The drawing under review shows one solid part. Ordinate dimensions are in mm from its lowest x, y, z. Coordinates: 2 decimals unless noted, no trailing zeros. Loops run counter-clockwise (first coordinate to the right, second up) from the corner with the lowest first, then second, coordinate; pieces in that order, holes last. Notation, with made-up numbers: (-39.75, 74.5) -> (4.25, 74.5) arc R10 ccw to (4.25, 81.5) -> close; hole circle Ø9 at (4, 45). An arc over 180 degrees is marked (long way). Use a Markdown table: item, result.
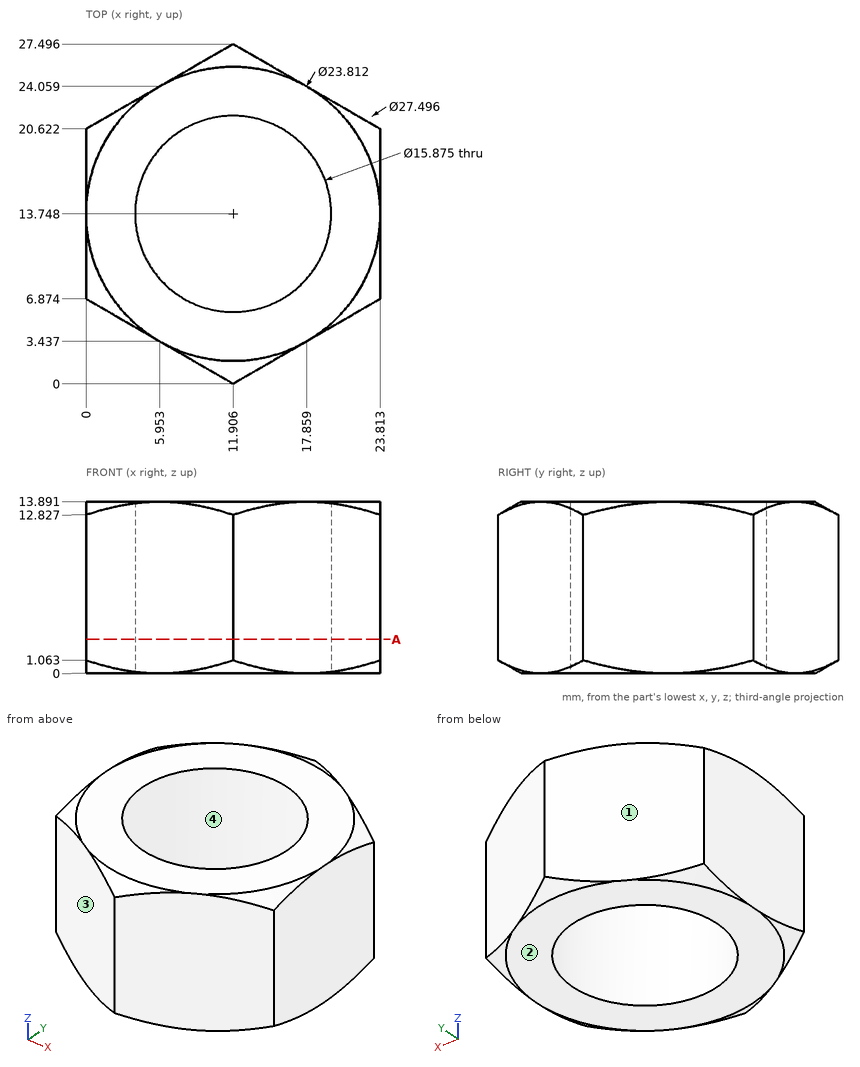
(1) For pin 1 Ø8 at (x, z) = (4, 6.5) entering from -Y (1 decimal); pin 2 Ø4 at (x, y) = (21, 16.5) entering from -Z; pin 3 Ø5 at (x, z) = (20, 12.5) entering from -Y; pin 4 Ø3 at (x, z) = (6.5, 4.5) entering from +Y, all flat-tipped, find the tip position at first contact; note any pin that passes through.
Found:
| item | result |
|---|---|
| pin 1 | stops at y = 2.3 |
| pin 2 | stops at z = 0 |
| pin 3 | stops at y = 3.23 |
| pin 4 | stops at y = 25.24 |
(2) Mouldability with a two-part tool opening along Y and no side actions: class the marked faces 1, 2, 3 and 4 as pulls with the +Y half, pulls with the -Y half, needs draft (parallel to the pull), parting line crosses it, or undercut.
Found:
| item | result |
|---|---|
| face 1 | pulls with the +Y half |
| face 2 | needs draft |
| face 3 | pulls with the -Y half |
| face 4 | undercut |
(3) For line 1 along Y through (x, z) = (16.75, 13.25) (1 decimal); line 2 along Y through (x, z) = (13.75, 11.75) (1 decimal); line 3 along X through (y, z) = (9.25, 12.5) (1 decimal), list the stretches that pass through material, from the lowest coordinate up.
Found:
| item | result |
|---|---|
| line 1 | y = 2.8 to 7.5, 20 to 24.7 |
| line 2 | y = 1.1 to 6, 21.5 to 26.4 |
| line 3 | x = 0 to 5.4, 18.4 to 23.8 |
(4) Take a section at A-A on z = 2.75. Write out the cut boundary in (x, y) (1 decimal).
Found:
| item | result |
|---|---|
| outline | (0, 6.9) -> (11.9, 0) -> (23.8, 6.9) -> (23.8, 20.6) -> (11.9, 27.5) -> (0, 20.6) -> close; hole circle Ø15.9 at (11.9, 13.7) |
